Geometry check sheet. Reference: the model listing, model coordinates, mm. Give positions to 0.01 mm unless a question says otherwise; leave off trailing zeros. Loops run counter-clockwise (first coordinate to the right, second up) from the corner with the lowest first, then second, coordinate; pieces in that order, holes last. Notation, with made-up numbers: (61.5, 46) - (69.5, 46) arc R18 ccw to (69.5, 52) - close; hole circle Ø5 at (70.5, 63.5). An arc over 180 degrees is marked (long way). Write item = value, one per line. Start each with the question number.
Autodesk Inventor part; units mm, degrees
ref_plane "YZ Plane" through (0, 0, 0) normal (1, 0, 0) x (0, 1, 0)
ref_plane "XZ Plane" through (0, 0, 0) normal (0, 1, 0) x (-1, 0, 0)
ref_plane "XY Plane" through (0, 0, 0) normal (0, 0, 1) x (1, 0, 0)
sketch "スケッチ1" plane through (0, 0, 0) normal (0, 1, 0) x (-1, 0, 0)
  line L0 (0, 0) -> (-35, 0)
  line L1 (-35, 0) -> (-35, -220)
  line L2 (-35, -220) -> (0, -220)
  line L3 (0, -220) -> (0, 0)
  arc A0 (-35, -220) -> (0, -220) centre (-17.5, -220) ccw
  dimension "d0" = 35
  dimension "d1" = 220
  dimension "d2" = 17.5
extrude "押し出し1" add sketch "スケッチ1" along normal blind 3
sketch "スケッチ2" plane through (0, 3, 0) normal (0, 1, 0) x (1, 0, 0)
  line L0 (0, 0) -> (35, 0) construction
  line L1 (17.5, 0) -> (17.5, 237.5) construction
  arc A0 (35, 220) -> (0, 220) centre (17.5, 220) ccw construction
hole "穴1" at (17.5, 3, -220) direction (0, -1, 0) diameter 8.5 end through all
sketch "スケッチ3" plane through (0, 3, 0) normal (0, 1, 0) x (1, 0, 0)
  circle A0 centre (17.5, 220) radius 4.25
  circle A1 centre (17.5, 220) radius 12.5
  point P0 (0, 0)
  point P1 (5, 220)
  point P2 (30, 220)
  point P3 (17.5, 232.5)
  point P4 (17.5, 207.5)
  dimension "d12" = 25
hole "穴2" at (5, 3, -220) at (30, 3, -220) at (17.5, 3, -232.5) at (17.5, 3, -207.5) direction (0, -1, 0) diameter 2.459 end through all
sketch "スケッチ4" plane through (0, 3, 0) normal (0, 1, 0) x (1, 0, 0)
  line L0 (0, 0) -> (35, 0) construction
  line L1 (17.5, 0) -> (17.5, 237.5) construction
  arc A0 (35, 220) -> (0, 220) centre (17.5, 220) ccw construction
  circle A1 centre (17.5, 220) radius 4.25
  point P0 (17.5, 137)
  point P1 (17.5, 127)
  point P2 (17.5, 117)
  point P3 (17.5, 107)
  point P4 (17.5, 97)
  point P5 (17.5, 87)
  point P6 (17.5, 77)
  point P7 (17.5, 67)
  point P8 (17.5, 57)
  point P9 (17.5, 47)
  point P10 (17.5, 37)
  point P11 (17.5, 27)
  point P12 (17.5, 17)
  point P13 (17.5, 7)
  dimension "d42" = 83
  dimension "d45" = 10
hole "穴3" at (17.5, 3, -137) at (17.5, 3, -127) at (17.5, 3, -117) at (17.5, 3, -107) at (17.5, 3, -97) at (17.5, 3, -87) at (17.5, 3, -77) at (17.5, 3, -67) at (17.5, 3, -57) at (17.5, 3, -47) at (17.5, 3, -37) at (17.5, 3, -27) at (17.5, 3, -17) at (17.5, 3, -7) direction (0, -1, 0) diameter 3.2 end through all
sketch "スケッチ5" plane through (0, 3, 0) normal (0, 1, 0) x (1, 0, 0)
  line L0 (0, 0) -> (35, 0) construction
  line L1 (17.5, 0) -> (17.5, 237.5) construction
  arc A0 (35, 220) -> (0, 220) centre (17.5, 220) ccw construction
  circle A1 centre (17.5, 137) radius 1.6 construction
  point P0 (17.5, 150)
  point P1 (17.5, 170)
  dimension "d50" = 13
  dimension "d51" = 20
hole "穴4" at (17.5, 3, -150) at (17.5, 3, -170) direction (0, -1, 0) diameter 6.6 end through all
sketch "スケッチ6" plane through (0, 3, 0) normal (0, 1, 0) x (1, 0, 0)
  line L0 (35, 0) -> (35, 220)
  line L1 (35, 204.2) -> (0, 204.2) construction
  line L2 (0, 220) -> (0, 0)
  circle A0 centre (17.5, 220) radius 4.25
  line L3 (17.5, 220) -> (17.5, 204.2) construction
  point P0 (28, 204.2)
  point P1 (7, 204.2)
  dimension "d52" = 15.8
  dimension "d53" = 10.5
  dimension "d54" = 10.5
hole "穴5" at (28, 3, -204.2) at (7, 3, -204.2) direction (0, -1, 0) diameter 3.3 end through all
properties part number "shoulder2_upper_plate" material "アルミニウム 5052"
1) Release check for a two-part mould opening along X. For faces 1 (the face through (15.27, 1.48, -152.43)), 2 (the face through (22, 3, -117)), 3 (the face through (17.4, 1.5, -173.3)), 4 (the face through (17.115, 1.479, -237.496)) record: pulls with the +X half, pulls with the -X half, needs draft (parallel to the pull), parting line crosses it, or undercut.
2) Cross-section at B-B on y = 1.75. Give the number of separate pieces and of enclosed holes in the cut face, and give its area (3 significant figures).
3) Gauge pin test, flat end, axial feed: P1, Ø1, axis at x = 31.5, y = 2.5, coming from the -Z side. Record the tip position at first contact, or that the pin passes through.
4) Cross-section at A-A on z = -150. Enter the section's corners in (x, y), and give its area (3 significant figures).
5) Material ranges on line 1 along X through (y, z) = (1, -220); line 2 along X through (y, z) = (1.4, -204.2); line 3 along Z through (x, y) = (29, 2.75), recorded low to high.
Checked values:
q1.face_1 = undercut
q1.face_2 = needs draft
q1.face_3 = undercut
q1.face_4 = parting line crosses it
q2.separate_pieces = 1
q2.enclosed_holes = 23
q2.area = 7,910 mm²
q3.P1 = -231.14
q4.outline = (0, 0) - (14.2, 0) - (14.2, 3) - (0, 3) - close; (20.8, 0) - (35, 0) - (35, 3) - (20.8, 3) - close
q4.area = 85.2 mm²
q5.line_1 = 0 to 3.77, 6.23 to 13.25, 21.75 to 28.77, 31.23 to 35
q5.line_2 = 0 to 5.35, 8.65 to 26.35, 29.65 to 35
q5.line_3 = -233.19 to -220.72, -219.28 to -205.51, -202.89 to 0
